Autodesk Inventor part; units mm, degrees
ref_plane "YZ Plane" through (0, 0, 0) normal (1, 0, 0) x (0, 1, 0)
ref_plane "XZ Plane" through (0, 0, 0) normal (0, 1, 0) x (-1, 0, 0)
ref_plane "XY Plane" through (0, 0, 0) normal (0, 0, 1) x (1, 0, 0)
sketch "Esboço1" plane through (0, 0, 0) normal (0, 0, 1) x (1, 0, 0)
  line L0 (-80, -50) -> (80, -50)
  line L1 (80, -50) -> (80, 50)
  line L2 (80, 50) -> (-80, 50)
  line L3 (-80, 50) -> (-80, -50)
  line L4 (-80, -50) -> (80, 50) construction
  line L5 (80, -50) -> (-80, 50) construction
  point P0 (0, 0)
  dimension "d0" = 100
  dimension "d1" = 160
extrude "Extrusão1" add sketch "Esboço1" along normal blind 20
sketch "Esboço2" plane through (0, 0, 20) normal (0, 0, 1) x (1, 0, 0)
  line L0 (-27.5, -40) -> (27.5, -40)
  line L1 (27.5, -40) -> (27.5, 40)
  line L2 (27.5, 40) -> (-27.5, 40)
  line L3 (-27.5, 40) -> (-27.5, -40)
  line L4 (-27.5, -40) -> (27.5, 40) construction
  line L5 (27.5, -40) -> (-27.5, 40) construction
  point P0 (0, 0)
  dimension "d4" = 55
  dimension "d5" = 80
extrude "Extrusão2" add sketch "Esboço2" along normal blind 110
fillet "Arredondamento1" radius 27.5 2 edges at (-27.5, 0, 130) (27.5, 0, 130)
sketch "Esboço3" plane through (-27.5, -40, 20) normal (0, -1, 0) x (1, 0, 0)
  arc A0 (55, 82.5) -> (0, 82.5) centre (27.5, 82.5) ccw
  point P0 (27.5, -20)
hole "Furo1" at (0, -40, 102.5) direction (0, 1, 0) diameter 30 end through all
sketch "Esboço4" plane through (-27.5, -40, 20) normal (-1, 0, 0) x (0, 0, 1)
  line L0 (20, 70) -> (50, 70)
  line L1 (50, 70) -> (50, 10)
  line L2 (50, 10) -> (20, 10)
  line L3 (20, 10) -> (20, 70)
  line L4 (20, 70) -> (50, 10) construction
  line L5 (50, 70) -> (20, 10) construction
  line L6 (-20, -10) -> (-20, 90)
  line L7 (82.5, 80) -> (82.5, 0)
  point P0 (-20, 40)
  point P1 (35, 40)
  point P2 (35, 40)
  point P3 (82.5, 40)
  dimension "d18" = 60
  dimension "d19" = 55
  dimension "d20" = 30
extrude "Extrusão3" cut sketch "Esboço4" against normal through all
sketch "Esboço5" plane through (0, 0, 20) normal (0, 0, 1) x (1, 0, 0)
  line L0 (-80, 50) -> (-80, -50)
  line L1 (-80, -50) -> (80, -50)
  line L2 (80, -50) -> (80, 50)
  point P0 (0, 0)
  point P1 (-60, 0)
  point P2 (60, 0)
  dimension "d23" = 20
  dimension "d24" = 50
  dimension "d25" = 20
  dimension "d26" = 50
hole "Furo2" at (-60, 0, 20) at (60, 0, 20) direction (0, 0, -1) diameter 20 end through all
fillet "Arredondamento2" radius 10 4 edges at (0, 30, 40) (0, -30, 70) (0, -30, 40) (0, 30, 70)
fillet "Arredondamento3" radius 10 2 edges at (-27.5, 0, 20) (27.5, 0, 20)
fillet "Arredondamento4" radius 20 4 edges at (80, -50, 10) (80, 50, 10) (-80, -50, 10) (-80, 50, 10)
equation "\"d8\" = 0.5 * d4"
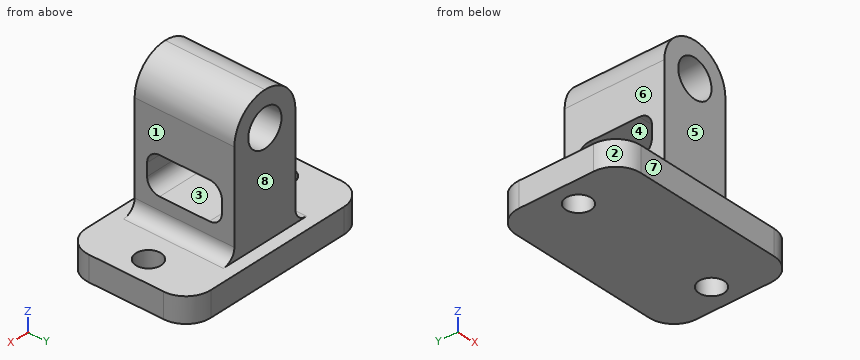
Verification items for the finished model (mm, model axes). Face numbers are marked on the shaded views. A direction names the side the tool comes from. Round coordinates to 2 decimals unless told otherwise and drop trailing zeros. Loops run counter-clockwise (first coordinate to the right, second up) from the corner with the lowest first, then second, coordinate; pieces in that order, holes last. Notation, with made-up numbers: (31, -17.5) - (48, -17.5) arc R17 ccw to (48, 13.5) - close; hole circle Ø5 at (-38.5, 29). An arc over 180 degrees is marked (long way). Answer in a Markdown table with one row per item. Add a question column.
Q1. Section check A-A on y = 0. State how many separate pieces and enclosed holes the cut face has, plus the area to 3 significant figures.
Q2. Section check D-D on x = -22. Enter the section's corners in (y, z).
Q3. Gauge pin test, flat ends, axial feed: pin 1 (5 mm diameter, centred on x = -1.5, z = 57.5, fed in from -Y); pin 2 (10 mm diameter, centred on y = -16.5, z = 82, fed in from -X); pin 3 (16 mm diameter, centred on x = -60, y = 0, fed in from -Z); pin 4 (5 mm diameter, centred on x = -9, z = 55, fed in from +Y). Record the tip position at first contact, or that the pin passes through.
Q4. Section check B-B on z = 9.5. Enter the section's corners in (x, y), plus the area to 3 significant figures.
Q5. Material ranges on line 1 (X direction, y = 0, z = 5.25); line 2 (Y direction, x = 60, z = 10); line 3 (Z direction, x = 0, y = -13.5), recorded low to high.
Q6. Release check for a two-part mould opening along Y. For the marked faces 1, 2 and 3 record: pulls with the +Y half, pulls with the -Y half, needs draft (parallel to the pull), parting line crosses it, or undercut.
Q7. Tool access check on the marked faces 4, 5, 6, 7 and 8. Record the directions out of +Z, -Z, +X, -X, +Y, -Y that give a thin tool (end or side, any length) a straight path to the whole face; none if there is none.
Found:
| question | item | result |
|---|---|---|
| 1 | separate pieces | 4 |
| 1 | enclosed holes | 1 |
| 1 | area | 5,810 mm² |
| 2 | outline | (-50, 0) - (50, 0) - (50, 20) - (40, 20) - (40, 119) - (-40, 119) - (-40, 20) - (-50, 20) - close; hole (-30, 50) arc R10 ccw to (-20, 40) - (20, 40) arc R10 ccw to (30, 50) - (30, 60) arc R10 ccw to (20, 70) - (-20, 70) arc R10 ccw to (-30, 60) - close |
| 3 | pin 1 | stops at y = -40 |
| 3 | pin 2 | stops at x = -27.5 |
| 3 | pin 3 | passes through |
| 3 | pin 4 | stops at y = 40 |
| 4 | outline | (-80, -30) arc R20 ccw to (-60, -50) - (60, -50) arc R20 ccw to (80, -30) - (80, 30) arc R20 ccw to (60, 50) - (-60, 50) arc R20 ccw to (-80, 30) - close; hole circle Ø20 at (-60, 0); hole circle Ø20 at (60, 0) |
| 4 | area | 15,000 mm² |
| 5 | line 1 | x = -80 to -70, -50 to 50, 70 to 80 |
| 5 | line 2 | y = -50 to -10, 10 to 50 |
| 5 | line 3 | z = 0 to 40, 70 to 87.5, 117.5 to 130 |
| 6 | face 1 | needs draft |
| 6 | face 2 | pulls with the -Y half |
| 6 | face 3 | undercut |
| 7 | face 4 | +X, -X |
| 7 | face 5 | +Z, +X, -X, -Y |
| 7 | face 6 | +Z, -X, +Y, -Y |
| 7 | face 7 | +Z, -Z, +X, -X, -Y |
| 7 | face 8 | +Z, +X, -X, +Y |
